from build123d import *

# Parameters (mm, degrees)
SKETCH015_W       = 111.7
SKETCH015_H       = 86.4
PAD007_DEPTH      = 1
SKETCH016_W       = 110.7
SKETCH016_H       = 85.4
PAD008_DEPTH      = 5.5
PAD005_DEPTH      = 55.85
PAD005_DEPTH_BACK = 55.85
PAD004_DEPTH      = 43.2
PAD004_DEPTH_BACK = 43.2


with BuildPart() as pad_bezel_lip:
    # Sketch015 → Pad007 (new body)
    with BuildSketch(Plane.XY):
        Rectangle(SKETCH015_W, SKETCH015_H)
    extrude(amount=-PAD007_DEPTH)


with BuildPart() as fusion_bezel_overlap:
    # Sketch016 → Pad008 (new body)
    with BuildSketch(Plane.XY):
        Rectangle(SKETCH016_W, SKETCH016_H)
    extrude(amount=PAD008_DEPTH)

    # Fusion002: union Pad (bezel lip)
    add(pad_bezel_lip.part)


with BuildPart() as pad_bezel_top_bottom:
    # Sketch006 → Pad005 (new body, two sides)
    with BuildSketch(Plane.YZ) as pad005_sk:
        Polygon((43.2, -1), (38.2, -1), (38.2, -0.6), (38.6, -0.6), (42.2, 4.5), (42.7, 4.5), (42.7, 0), (43.2, 0), align=None)
        Polygon((-38.6, -0.6), (-42.2, 4.5), (-42.7, 4.5), (-42.7, 0), (-43.2, 0), (-43.2, -1), (-38.2, -1), (-38.2, -0.6), align=None)
    extrude(amount=PAD005_DEPTH)
    extrude(pad005_sk.sketch, amount=-PAD005_DEPTH_BACK)


with BuildPart() as common:
    # Sketch005 → Pad004 (new body, two sides)
    with BuildSketch(Plane.XZ) as pad004_sk:
        Polygon((-55.85, -1), (-50.85, -1), (-50.85, -0.6), (-51.25, -0.6), (-54.85, 4.5), (-55.35, 4.5), (-55.35, 0), (-55.85, 0), align=None)
        Polygon((50.85, -1), (55.85, -1), (55.85, 0), (55.35, 0), (55.35, 4.5), (54.85, 4.5), (51.25, -0.6), (50.85, -0.6), align=None)
    extrude(amount=PAD004_DEPTH)
    extrude(pad004_sk.sketch, amount=-PAD004_DEPTH_BACK)

    # Fusion: union Pad (bezel top/bottom)
    add(pad_bezel_top_bottom.part)

    # Common: intersect Fusion (bezel overlap)
    add(fusion_bezel_overlap.part, mode=Mode.INTERSECT)


with BuildPart() as common_1:
    # Common placement: moved
    add(common.part.moved(Location((0, 11, 0))))


solid = common_1.part
Input: part model. Units: mm. Frame: model coordinates. A direction names the side the tool comes from. Give positions to 0.01 mm unless a question says otherwise; leave off trailing zeros. Order: outer loops, then holes, each group sorted by start corner. A loop starts at its lowest first (then second) coordinate and runs counter-clockwise, first axis right, second up. Notation, with made-up numbers: (3.25, 78) - (16.25, 78) arc R18 ccw to (16.25, 98) - close; hole circle Ø4 at (-33.75, 59). An arc over 180 degrees is marked (long way). Answer as a JSON object with one key per item and string values. Group by question number.
Q1. First-contact query: pin 1 Ø1.3 at (y, z) = (-2.5, 1.5) entering from -X; pin 2 Ø1.3 at (x, z) = (-21, 2) entering from +Y; pin 3 Ø1.3 at (y, z) = (-7.5, 1.5) entering from +X. Flat tips, straight axial feed; report the tip coordinate or a pass-through.
Q2. Cut plane C-C, the plane x = -47.5. Output: boundary loops of the cut face in (y, z), then the cut area to 3 significant figures.
Q3. Line query: probe 1 along Z at (x, y) = (51, 22); probe 2 along X at (y, z) = (-3.5, 2.3); probe 3 along Y at (x, z) = (28.5, 1.4). Output: solid intervals per line, ascending.
Q4. Set-up query: faces 4 (the face through (-55.35, 10, 2)), 5 (the face through (-1, 53.7, 2)), 6 (the face through (0.77, -29.37, 1.91)). Return all of +Z, -Z, +X, -X, +Y, -Y with unobstructed straight access to the full face (end or side cutting, diameter ignored); none if empty.
Q5. Mould query, pull axis X, two halves, no side actions, for faces 1 (the face through (55.35, 10, 2)), 2 (the face through (0.77, 51.37, 1.91)), 3 (the face through (-1, -31.7, 2)). Classes: pulls with the +X half, pulls with the -X half, needs draft (parallel to the pull), parting line crosses it, or undercut.
Q6. Cut plane A-A, the plane z = 1.95. Output: boundary loops of the cut face in (x, y).
Q7. Cut plane B-B, the plane y = 17. Output: boundary loops of the cut face in (x, z), then the cut area to 3 significant figures.
Results:
{
 "1": {"pin 1": "x = -55.35", "pin 2": "y = 53.7", "pin 3": "x = 55.35"},
 "2": {"outline": "(-32.2, -1) - (-27.2, -1) - (-27.2, -0.6) - (-27.6, -0.6) - (-31.2, 4.5) - (-31.7, 4.5) - (-31.7, 0) - (-32.2, 0) - close; (49.2, -1) - (54.2, -1) - (54.2, 0) - (53.7, 0) - (53.7, 4.5) - (53.2, 4.5) - (49.6, -0.6) - (49.2, -0.6) - close", "area": "28.1 mm^2"},
 "3": {"probe 1": "-1 to -0.6", "probe 2": "-55.35 to -53.3, 53.3 to 55.35", "probe 3": "-31.7 to -29.01, 51.01 to 53.7"},
 "4": {"face 4": "+Z, -X, +Y, -Y", "face 5": "+Z, +X, -X, +Y", "face 6": "+Z"},
 "5": {"face 1": "pulls with the +X half", "face 2": "undercut", "face 3": "needs draft"},
 "6": {"outline": "(-55.35, -31.7) - (55.35, -31.7) - (55.35, 53.7) - (-55.35, 53.7) - close; hole (-53.05, -29.4) - (53.05, -29.4) - (53.05, 51.4) - (-53.05, 51.4) - close"},
 "7": {"outline": "(-55.85, -1) - (-50.85, -1) - (-50.85, -0.6) - (-51.25, -0.6) - (-54.85, 4.5) - (-55.35, 4.5) - (-55.35, 0) - (-55.85, 0) - close; (50.85, -1) - (55.85, -1) - (55.85, 0) - (55.35, 0) - (55.35, 4.5) - (54.85, 4.5) - (51.25, -0.6) - (50.85, -0.6) - close", "area": "28.1 mm^2"}
}
